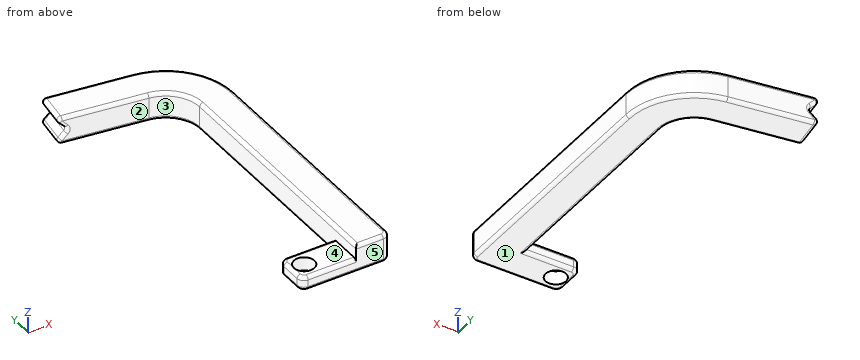
```python
from build123d import *

# Parameters (mm, degrees)
EXTRUDE_1_DEPTH     = 2
EXTRUDE_2_DEPTH     = 2
CUT_EXTRUDE_1_DEPTH = 5
SKETCH_4_R          = 1.5
CUT_EXTRUDE_2_DEPTH = 48.894743495
FILLET_1_R          = 0.5


with BuildPart() as part:
    # 草图1 → 凸台-拉伸1 (new body)
    with BuildSketch(Plane.XY):
        with BuildLine():
            Line((-5.5, 2.5), (5.5, 2.5))
            ThreePointArc((5.5, 2.5), (6.207106781, 2.207106781), (6.5, 1.5))
            Line((6.5, 1.5), (6.5, -1.5))
            ThreePointArc((6.5, -1.5), (6.207106781, -2.207106781), (5.5, -2.5))
            Line((5.5, -2.5), (-5.5, -2.5))
            ThreePointArc((-5.5, -2.5), (-6.207106781, -2.207106781), (-6.5, -1.5))
            Line((-6.5, -1.5), (-6.5, 1.5))
            ThreePointArc((-6.5, 1.5), (-6.207106781, 2.207106781), (-5.5, 2.5))
        make_face()
    extrude(amount=EXTRUDE_1_DEPTH)

    # 草图2 → 凸台-拉伸2 (add, symmetric)
    with BuildSketch(Plane.XY.offset(2)):
        with BuildLine():
            Line((6.5, 1.5), (6.5, 33.5))
            ThreePointArc((6.5, 33.5), (4.047095802, 40.06059029), (-2.10826899, 43.402680687))
            Line((-2.10826899, 43.402680687), (-14.981753884, 45.211931))
            Line((-14.981753884, 45.211931), (-15.677619389, 40.260590656))
            Line((-15.677619389, 40.260590656), (-2.804134495, 38.451340344))
            ThreePointArc((-2.804134495, 38.451340344), (0.273547901, 36.780295145), (1.5, 33.5))
            Line((1.5, 33.5), (1.5, 2.5))
            Line((1.5, 2.5), (1.5, -2.5))
            Line((1.5, -2.5), (5.5, -2.5))
            ThreePointArc((5.5, -2.5), (6.207106781, -2.207106781), (6.5, -1.5))
            Line((6.5, -1.5), (6.5, 1.5))
        make_face()
    extrude(amount=EXTRUDE_2_DEPTH, both=True)

    # 草图3 → 切除-拉伸1 (cut)
    with BuildSketch(Plane(origin=(5.940864687, 42.271448722, 0), x_dir=(0.9902680687415704, -0.13917310096006608, 0), z_dir=(0.13917310096006608, 0.9902680687415704, 0))):
        Polygon((-21.128237123, 0), (-19.126013359, -2), (-21.128237123, -4), align=None)
    extrude(amount=-CUT_EXTRUDE_1_DEPTH, mode=Mode.SUBTRACT)

    # 草图4 → 切除-拉伸2 (cut, through all)
    with BuildSketch(Plane.XY.offset(2)):
        with Locations((-4.5, 0)):
            Circle(SKETCH_4_R)
    extrude(amount=-CUT_EXTRUDE_2_DEPTH, mode=Mode.SUBTRACT)

    # 圆角1
    fillet_1_edges = [part.edges().sort_by_distance(p)[0] for p in [
        (-6.5, 0, 0),
        (-6.207106781, 2.207106781, 0),
        (-6.207106781, 2.207106781, 2),
        (-6.5, 0, 2),
        (-6.207106781, -2.207106781, 2),
        (-2, -2.5, 2),
        (-2, 2.5, 0),
        (-2, 2.5, 2),
        (1.5, 18, 0),
        (4.047095802, 40.06059029, 0),
        (-8.545011437, 44.307305844, 0),
        (-15.329686636, 42.736260828, 0),
        (-9.240876942, 39.3559655, 0),
        (0.273547901, 36.780295145, 0),
        (6.5, 16, 4),
        (4.047095802, 40.06059029, 4),
        (-8.545011437, 44.307305844, 4),
        (-15.329686636, 42.736260828, 4),
        (-9.240876942, 39.3559655, 4),
        (0.273547901, 36.780295145, 4),
        (1.5, 15.5, 4),
        (3.5, -2.5, 4),
        (6.207106781, -2.207106781, 4),
        (-13.346948377, 42.457605138, 2),
        (-13.990384754, 45.072603155, 3),
        (-13.990384754, 45.072603155, 1),
        (-14.686250259, 40.121262811, 1),
        (-14.686250259, 40.121262811, 3),
        (6.5, 16, 0),
        (6.207106781, -2.207106781, 0),
        (0, -2.5, 0),
        (-6.207106781, -2.207106781, 0),
    ]]
    fillet(fillet_1_edges, radius=FILLET_1_R - 0.0001)  # a hair under: the kernel refuses the full size


solid = part.part
```
Could you check a few things on this model? Use its own coordinates, in mm. Face numbers are marked on the shaded views. A direction names the side the tool comes from. Round coordinates to 2 decimals unless told otherwise and drop trailing zeros. Write each loop counter-clockwise with the first axis right and the second up, starting at its lowest first coordinate (ties: lowest second). Pieces come first, ordered by that corner, then holes. Notation, with made-up numbers: M -35,29 L -7,29 A17 ccw -7,45 Z; hole C 23,35 d5. An arc over 180 degrees is marked long. Answer in a Markdown table with one row per item. Add a question column.
Q1. Will these pins go through, and if not, where does the flat tip stop? pin 1 Ø3.5 at (x, y) = (-4.5, 0) entering from +Z; pin 2 Ø1.1 at (y, z) = (0.5, 1) entering from -X; pin 3 Ø0.9 at (y, z) = (23.5, 2) entering from -X.
Q2. If we mould it in two halves opening along Y, with no side actions, what happens to the marked faces 3, 4 and 5? For each: +Y half, -Y half, draft (parallel to the pull), parting line (faces both ways), or undercut.
Q3. On a 3-axis mill with a long thin cutter (end or side, diameter ignored), from which of +Z, -Z, +X, -X, +Y, -Y can I reach the whole of each face in a straight line? I mean the marked faces 1 and 2. Say none if no direction works.
Q4. If I drill on line 1 (Y direction, x = -4.5, z = 1); line 2 (X direction, y = 13.5, z = 0.8); line 3 (Z direction, x = 1, y = 0.5), over which ranges is the centre line in solid material (lowest first)? Write a range as from..to.
Q5. Imagine slicing it at C-C (x = -4.25). Give the number of separate pieces and of enclosed holes in the cut face, then the cut area to 3 significant figures.
Q6. Imagine slicing it at B-B (y = 14). Please give me the cut outline in (x, z), then the cut area to 3 significant figures.
Values:
| question | item | result |
|---|---|---|
| 1 | pin 1 | z = 2 |
| 1 | pin 2 | x = -6.5 |
| 1 | pin 3 | x = 1.5 |
| 2 | face 3 | undercut |
| 2 | face 4 | draft |
| 2 | face 5 | -Y half |
| 3 | face 1 | -Z, +X, -X, +Y, -Y |
| 3 | face 2 | +Z, -Z, -X |
| 4 | line 1 | -2.5..-1.5, 1.5..2.5, 38.69..43.74 |
| 4 | line 2 | 1.5..6.5 |
| 4 | line 3 | 0..2 |
| 5 | separate pieces | 3 |
| 5 | enclosed holes | 0 |
| 5 | area | 23.8 mm^2 |
| 6 | outline | M 1.5,0.5 A0.5 ccw 2,0 L 6,0 A0.5 ccw 6.5,0.5 L 6.5,3.5 A0.5 ccw 6,4 L 2,4 A0.5 ccw 1.5,3.5 Z |
| 6 | area | 19.8 mm^2 |
